The figure shows three views and two pictorial views of one solid part (mm, origin at its lowest corner). Answer the questions. A direction names the side the tool comes from. Round coordinates to 2 decimals unless told otherwise and drop trailing zeros. Write each loop counter-clockwise with the first axis right and the second up, starting at its lowest first coordinate (ties: lowest second). Pieces come first, ordered by that corner, then holes.
Item 1: Find the intervals of material crossed by probe 1 along Y at (x, z) = (16, 7.75); probe 2 along Z at (x, y) = (4.5, 1.35); probe 3 along X at (y, z) = (21.5, 9), in increasing order.
Item 2: For a pull along Y with two mould halves and no side action, classify the marked faces 6, 7 and 8 as +Y half, -Y half, draft (parallel to the pull), parting line (faces both ways), or undercut.
Item 3: Each of these flat-tipped pins is pushed along its axis until it touches: pin 1 (12 mm diameter, centred on x = 30.5, y = 17, fed in from -Z); pin 2 (1.8 mm diameter, centred on x = 4.5, z = 8, fed in from -Y); pin 3 (3 mm diameter, centred on y = 21.5, z = 10.5, fed in from -X); pin 4 (4 mm diameter, centred on x = 5.5, z = 9.5, fed in from +Y). Where does it stop, or does it pass through?
Item 4: Find section C-C on x = 4.5. Give the vertices of the cut face in (y, z), then the cut area to 3 significant figures.
Item 5: Find section D-D on z = 3. Give the vertices of the cut face in (x, y), then the cut area to 4 significant figures.
Item 6: Find section B-B on x = 41. Give the vertices of the cut face in (y, z).
Item 7: Find section A-A on z = 8. Give the vertices of the cut face in (x, y).
Item 8: A tool of negligible diameter and unlimited length cuts with its end or side. For the marked faces 1, 2, 3, 4 and 5, from which of +Z, -Z, +X, -X, +Y, -Y can it reach the whole face along a straight path? Write none if from no direction.
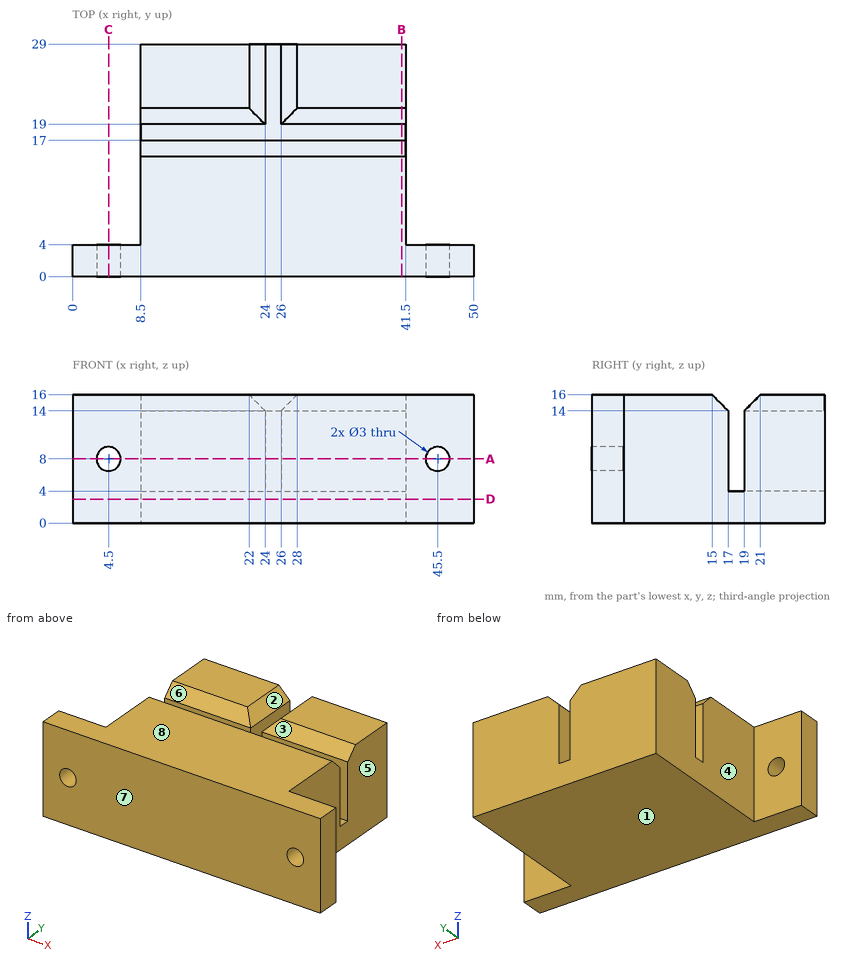
Check values:
1. probe 1: y = 0 to 17, 19 to 29
1. probe 2: z = 0 to 6.5, 9.5 to 16
1. probe 3: x = 8.5 to 24, 26 to 41.5
2. face 6: undercut
2. face 7: -Y half
2. face 8: draft
3. pin 1: stops at z = 0
3. pin 2: passes through
3. pin 3: stops at x = 8.5
3. pin 4: stops at y = 4
4. outline: (0, 0) - (4, 0) - (4, 6.5) - (0, 6.5) - close; (0, 9.5) - (4, 9.5) - (4, 16) - (0, 16) - close
4. area: 52.0 mm2
5. outline: (0, 0) - (50, 0) - (50, 4) - (41.5, 4) - (41.5, 29) - (8.5, 29) - (8.5, 4) - (0, 4) - close
5. area: 1,025 mm2
6. outline: (0, 0) - (29, 0) - (29, 16) - (21, 16) - (19, 14) - (19, 4) - (17, 4) - (17, 14) - (15, 16) - (0, 16) - close
7. outline: (0, 0) - (3, 0) - (3, 4) - (0, 4) - close; (6, 0) - (44, 0) - (44, 4) - (41.5, 4) - (41.5, 17) - (8.5, 17) - (8.5, 4) - (6, 4) - close; (8.5, 19) - (24, 19) - (24, 29) - (8.5, 29) - close; (26, 19) - (41.5, 19) - (41.5, 29) - (26, 29) - close; (47, 0) - (50, 0) - (50, 4) - (47, 4) - close
8. face 1: -Z, +X, -X, +Y, -Y
8. face 2: +Z, +Y
8. face 3: +Z, +X, -X
8. face 4: +Z, -Z, -X, +Y
8. face 5: +Z, -Z, +X, +Y
